Input: part model. Units: mm. Frame: model coordinates. Face numbers are marked on the shaded views. A direction names the side the tool comes from. Coordinates: 2 decimals unless noted, no trailing zeros. Loops run counter-clockwise (first coordinate to the right, second up) from the corner with the lowest first, then second, coordinate; pieces in that order, holes last.
Item 1: Section D-D on y = 43.5. Return loops of the section in (x, z).
Item 2: Section A-A on x = 0. Return loops of the section in (y, z).
Item 3: Section C-C on y = -20. Return loops of the section in (x, z), and give its area (3 significant figures).
Item 4: Ray query, line 1 along Y through (x, z) = (0.5, 0); line 2 along Z through (x, y) = (0.5, -30); line 3 along Z through (x, y) = (1.25, -30). Return the intervals inside material, ascending.
Item 5: Reachability of the marked faces 1 and 2 from +Z, -Z, +X, -X, +Y, -Y: full face, straight path, thin tool, end or side. Return the list, or none.
Item 6: Contact query for flat-ended pins moving along their axis: P1, Ø10, axis at x = 4.5, z = -7, coming from the -Y side; P2, Ø12, axis at y = -4.5, z = 12, coming from the -X side; P3, Ø10, axis at y = 12.5, z = -2.5, coming from the +X side; P4, Ø6, axis at x = 3, y = -27, coming from the -Z side. Output: stop coordinate, or through.
Item 7: Section B-B on y = -30. Return loops of the section in (x, z).
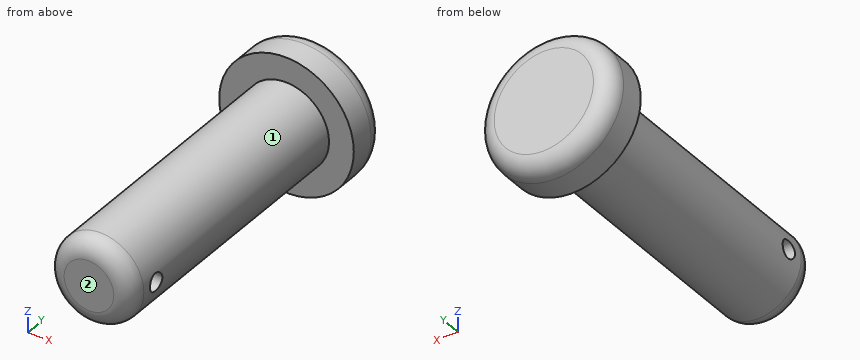
```python
from build123d import *

# Parameters (mm, degrees)
SKETCH5_R          = 2.5
CUT_EXTRUDE1_DEPTH = 35


with BuildPart() as part:
    # Sketch1 → Revolve3 (revolve)
    with BuildSketch(Plane.XY):
        with BuildLine():
            Line((0, 52), (14, 52))
            ThreePointArc((14, 52), (17.535533906, 50.535533906), (19, 47))
            Line((19, 47), (19, 40))
            Line((19, 40), (12, 40))
            Line((12, 40), (12, -35))
            ThreePointArc((12, -35), (10.535533906, -38.535533906), (7, -40))
            Line((7, -40), (0, -40))
            Line((0, -40), (0, 52))
        make_face()
    revolve(axis=Axis((0, 87.076923077, 0), (0, -1, 0)))

    # Sketch5 → Cut-Extrude1 (cut, symmetric)
    with BuildSketch(Plane(origin=(0, 0, 0), x_dir=(0, 0, -1), z_dir=(1, 0, 0))):
        with Locations((0, -30)):
            Circle(SKETCH5_R)
    extrude(amount=CUT_EXTRUDE1_DEPTH, both=True, mode=Mode.SUBTRACT)


solid = part.part
```
Results found:
1. outline: circle Ø38 at (0, 0)
2. outline: (-40, -7) arc R5 ccw to (-35, -12) - (40, -12) - (40, -19) - (47, -19) arc R5 ccw to (52, -14) - (52, 14) arc R5 ccw to (47, 19) - (40, 19) - (40, 12) - (-35, 12) arc R5 ccw to (-40, 7) - close; hole circle Ø5 at (-30, 0)
3. outline: circle Ø24 at (0, 0)
3. area: 452 mm2
4. line 1: y = -40 to -32.5, -27.5 to 52
4. line 2: z = -11.99 to -2.5, 2.5 to 11.99
4. line 3: z = -11.93 to -2.5, 2.5 to 11.93
5. face 1: -Y
5. face 2: +Z, -Z, +X, -X, -Y
6. P1: stops at y = -40
6. P2: stops at x = -10.39
6. P3: stops at x = 12
6. P4: stops at z = -12
7. outline: (-11.74, -2.5) arc R12 ccw to (11.74, -2.5) - close; (-11.74, 2.5) - (11.74, 2.5) arc R12 ccw to start
